from build123d import *

# Parameters (mm, degrees)
BOSS_EXTRUDE1_DEPTH = 125
CUT_EXTRUDE1_REACH  = 139.298
SKETCH2_R           = 2.665
CUT_EXTRUDE2_REACH  = 139.298
SKETCH3_R           = 5


with BuildPart() as part:
    # Sketch1 → Boss-Extrude1 (new body)
    with BuildSketch(Plane.XY):
        Polygon((0, 0), (0, 50.8), (-25.4, 50.8), (-25.4, 47.625), (-3.175, 47.625), (-3.175, 0), align=None)
    extrude(amount=BOSS_EXTRUDE1_DEPTH)

    # Sketch2 → Cut-Extrude1 (cut, up to next)
    with BuildSketch(Plane(origin=(0, 0, 0), x_dir=(0, 0, -1), z_dir=(1, 0, 0)), mode=Mode.PRIVATE) as cut_extrude1_sk1:
        with Locations((-115, 10)):
            Circle(SKETCH2_R)
    cut_extrude1_tool1 = extrude(cut_extrude1_sk1.sketch, amount=-CUT_EXTRUDE1_REACH, mode=Mode.PRIVATE) & part.part
    # Sketch2 → Cut-Extrude1 (cut, up to next)
    with BuildSketch(Plane(origin=(0, 0, 0), x_dir=(0, 0, -1), z_dir=(1, 0, 0)), mode=Mode.PRIVATE) as cut_extrude1_sk2:
        with Locations((-10, 10)):
            Circle(SKETCH2_R)
    cut_extrude1_tool2 = extrude(cut_extrude1_sk2.sketch, amount=-CUT_EXTRUDE1_REACH, mode=Mode.PRIVATE) & part.part
    # Sketch2 → Cut-Extrude1 (cut, up to next)
    with BuildSketch(Plane(origin=(0, 0, 0), x_dir=(0, 0, -1), z_dir=(1, 0, 0)), mode=Mode.PRIVATE) as cut_extrude1_sk3:
        with Locations((-62.5, 10)):
            Circle(SKETCH2_R)
    cut_extrude1_tool3 = extrude(cut_extrude1_sk3.sketch, amount=-CUT_EXTRUDE1_REACH, mode=Mode.PRIVATE) & part.part
    add(cut_extrude1_tool1.solids().sort_by_distance((0, 10, 115))[0], mode=Mode.SUBTRACT)
    add(cut_extrude1_tool2.solids().sort_by_distance((0, 10, 10))[0], mode=Mode.SUBTRACT)
    add(cut_extrude1_tool3.solids().sort_by_distance((0, 10, 62.5))[0], mode=Mode.SUBTRACT)

    # Sketch3 → Cut-Extrude2 (cut, up to next)
    with BuildSketch(Plane(origin=(0, 50.8, 0), x_dir=(1, 0, 0), z_dir=(0, 1, 0)), mode=Mode.PRIVATE) as cut_extrude2_sk1:
        with Locations(Location((-13.675, -112.5, 0), (0, 0, 270))):
            Circle(SKETCH3_R)
    cut_extrude2_tool1 = extrude(cut_extrude2_sk1.sketch, amount=-CUT_EXTRUDE2_REACH, mode=Mode.PRIVATE) & part.part
    # Sketch3 → Cut-Extrude2 (cut, up to next)
    with BuildSketch(Plane(origin=(0, 50.8, 0), x_dir=(1, 0, 0), z_dir=(0, 1, 0)), mode=Mode.PRIVATE) as cut_extrude2_sk2:
        with BuildLine():
            ThreePointArc((-8.675, -12.5), (-10.139466094, -8.964466094), (-13.675, -7.5))
            ThreePointArc((-13.675, -7.5), (-18.675, -12.5), (-13.675, -17.5))
            ThreePointArc((-13.675, -17.5), (-10.139466094, -16.035533906), (-8.675, -12.5))
        make_face()
    cut_extrude2_tool2 = extrude(cut_extrude2_sk2.sketch, amount=-CUT_EXTRUDE2_REACH, mode=Mode.PRIVATE) & part.part
    add(cut_extrude2_tool1.solids().sort_by_distance((-13.675, 50.8, 112.5))[0], mode=Mode.SUBTRACT)
    add(cut_extrude2_tool2.solids().sort_by_distance((-13.675, 50.8, 12.5))[0], mode=Mode.SUBTRACT)


solid = part.part
Geometry check sheet. Reference: the model listing, model coordinates, mm. A direction names the side the tool comes from. Give positions to 0.01 mm unless a question says otherwise; leave off trailing zeros. Write each loop counter-clockwise with the first axis right and the second up, starting at its lowest first coordinate (ties: lowest second). Pieces come first, ordered by that corner, then holes. Notation, with made-up numbers: M 32.25,84.5 L 74.25,84.5 A12 cw 74.25,95.5 Z; hole C 12.25,42 d4. An arc over 180 degrees is marked long. Answer as CSV lines item,"result". Start each with the question number.
Q1. Section check A-A, the plane y = 10. Record the cut outline in (x, z) (3 decimals).
Q2. Go/stop test with flat-tipped pins: pin 1 (6 mm diameter, centred on y = 39.5, z = 79.5, fed in from +X); pin 2 (4.5 mm diameter, centred on y = 10, z = 10, fed in from -X); pin 3 (5 mm diameter, centred on x = -7, z = 43.5, fed in from -Y) (3 decimals); pin 4 (5 mm diameter, centred on y = 20.5, z = 37.5, fed in from -X) (3 decimals). Record where each tip stops, or that it passes through.
Q3. Section check B-B, the plane z = 14. Record the cut outline in (x, y) (3 decimals), then the cut area to 3 significant figures.
Q4. Tool access check on faces 5 (the face through (-2, 35, 125)), 6 (the face through (-14, 47.625, 62)). Record the directions out of +Z, -Z, +X, -X, +Y, -Y that give a thin tool (end or side, any length) a straight path to the whole face; none if there is none.
Q5. Section check C-C, the plane x = -12. Record the cut outline in (y, z) (3 decimals), then the cut area to 3 significant figures.
Q6. Release check for a two-part mould opening along Y. For faces 1 (the face through (-13, 50.8, 62)), 2 (the face through (-25.4, 49, 62)), 3 (the face through (-1.57, 10.8, 112.46)), 4 (the face through (-2, 0, 62)) record: pulls with the +Y half, pulls with the -Y half, needs draft (parallel to the pull), parting line crosses it, or undercut.
Q7. Section check D-D, the plane z = 115. Record the cut outline in (x, y) (3 decimals), then the cut area to 3 significant figures.
Q8. Material ranges on L1, parallel to X at y = 50.15, z = 112.5 (3 decimals); L2, parallel to Y at x = -1.6, z = 10 (3 decimals); L3, parallel to X at y = 48, z = 112, recorded low to high.
Geometry says:
1,outline,"M -3.175,0 L 0,0 L 0,7.335 L -3.175,7.335 Z; M -3.175,12.665 L 0,12.665 L 0,59.835 L -3.175,59.835 Z; M -3.175,65.165 L 0,65.165 L 0,112.335 L -3.175,112.335 Z; M -3.175,117.665 L 0,117.665 L 0,125 L -3.175,125 Z"
2,pin 1,"x = 0"
2,pin 2,"through"
2,pin 3,"y = 47.625"
2,pin 4,"x = -3.175"
3,outline,"M -25.4,47.625 L -18.445,47.625 L -18.445,50.8 L -25.4,50.8 Z; M -8.905,47.625 L -3.175,47.625 L -3.175,0 L 0,0 L 0,50.8 L -8.905,50.8 Z"
3,area,"202 mm^2"
4,face 5,"+Z, +X, -X, +Y, -Y"
4,face 6,"+Z, -Z, -X, -Y"
5,outline,"M 47.625,0 L 50.8,0 L 50.8,7.789 L 47.625,7.789 Z; M 47.625,17.211 L 50.8,17.211 L 50.8,107.789 L 47.625,107.789 Z; M 47.625,117.211 L 50.8,117.211 L 50.8,125 L 47.625,125 Z"
5,area,"337 mm^2"
6,face 1,"pulls with the +Y half"
6,face 2,"needs draft"
6,face 3,"undercut"
6,face 4,"pulls with the -Y half"
7,outline,"M -25.4,47.625 L -18.005,47.625 L -18.005,50.8 L -25.4,50.8 Z; M -9.345,47.625 L -3.175,47.625 L -3.175,12.665 L 0,12.665 L 0,50.8 L -9.345,50.8 Z; M -3.175,0 L 0,0 L 0,7.335 L -3.175,7.335 Z"
7,area,"187 mm^2"
8,L1,"-25.4 to -18.675, -8.675 to 0"
8,L2,"0 to 7.335, 12.665 to 50.8"
8,L3,"-25.4 to -18.65, -8.7 to 0"
